```python
from build123d import *

# Parameters (mm, degrees)
F3_DEPTH = 35.967948
F5_COUNT = 3
F5_ANGLE = 240
F9_COUNT = 3
F9_ANGLE = 240


with BuildPart() as f1:
    # F0 (on Front) → F1 (revolve)
    with BuildSketch(Plane.XZ):
        with BuildLine():
            Line((-35.966948, -26.884749), (-31.12, -26.884749))
            Line((-31.12, -26.884749), (-31.12, -6.884749))
            Line((-31.12, -6.884749), (-25, 13.115251))
            Line((-25, 13.115251), (-6.375, 13.115251))
            Line((-6.375, 13.115251), (-6.375, 33.962199))
            Line((-6.375, 33.962199), (-11.221948, 33.962199))
            ThreePointArc((-11.221948, 33.962199), (-15.908239, 22.64849), (-27.221948, 17.962199))
            Line((-27.221948, 17.962199), (-28.585629, 17.962199))
            Line((-28.585629, 17.962199), (-35.966948, -6.159757))
            Line((-35.966948, -6.159757), (-35.966948, -26.884749))
        make_face()
    revolve(axis=Axis((0, 0, 3.115251), (0, 0, -1)))

    # F2 (on Front) → F3 (cut, through all)
    with BuildSketch(Plane.XZ):
        with BuildLine():
            ThreePointArc((5.600963, 5.956731), (0.100963, 11.456731), (-5.399037, 5.956731))
            Line((-5.399037, 5.956731), (5.600963, 5.956731))
        make_face()
        with BuildLine():
            Line((5.600963, 5.956731), (-5.399037, 5.956731))
            ThreePointArc((-5.399037, 5.956731), (0.100963, 0.456731), (5.600963, 5.956731))
        make_face()
    extrude(amount=-F3_DEPTH, mode=Mode.SUBTRACT)


with BuildPart() as f5_1:
    # F5: instance of F1
    add(f1.part.rotate(Axis((0, 0, 22.867789), (0, 0, 1)), 1 * F5_ANGLE / (F5_COUNT - 1)))


with BuildPart() as f5_2:
    # F5: instance of F1
    add(f1.part.rotate(Axis((0, 0, 22.867789), (0, 0, 1)), 2 * F5_ANGLE / (F5_COUNT - 1)))


with BuildPart() as f9_1:
    # F9: instance of F1
    add(f1.part.rotate(Axis((0, 0, 23.663558), (0, 0, 1)), 1 * F9_ANGLE / (F9_COUNT - 1)))


with BuildPart() as f9_2:
    # F9: instance of F1
    add(f1.part.rotate(Axis((0, 0, 23.663558), (0, 0, 1)), 2 * F9_ANGLE / (F9_COUNT - 1)))


solid = f1.part
```
Input: part model. Units: mm. Frame: model coordinates. A direction names the side the tool comes from. Coordinates: 2 decimals unless noted, no trailing zeros. Loops run counter-clockwise (first coordinate to the right, second up) from the corner with the lowest first, then second, coordinate; pieces in that order, holes last. Notation, with made-up numbers: M 42,37 L 53,37 A18 ccw 53,64 Z; hole C 2,33.25 d6. An arc over 180 degrees is marked long. One line per item, written item: value.
(1) Section C-C (z = -19). Output: boundary loops of the cut face in (x, y), and give its area (3 significant figures).
Filled in:
outline: C 0,0 d71.93; hole C 0,0 d62.24
area: 1,020 mm^2
(2) Section D-D (z = 30.5). Output: boundary loops of the cut face in (x, y) (3 decimals).
Filled in:
outline: C 0,0 d23.202; hole C 0,0 d12.75
(3) Line query: line 1 along Y through (x, z) = (0, -14); line 2 along X through (y, z) = (-1.5, -9.5); line 3 along Y through (x, z) = (-2, -11). Output: solid intervals per line, ascending. Write a range as from..to.
Filled in:
line 1: -35.97..-31.12, 31.12..35.97
line 2: -35.94..-31.08, 31.08..35.94
line 3: -35.91..-31.06, 31.06..35.91
(4) Pull-direction query (Y, two-part tool) for faces 1 (the flat face through (-5, -5, 13.115)), 2 (the conical face through (6.47, -29.16, 13.77)), 3 (the flat face through (5, -5, 33.962)); classes: +Y half, -Y half, draft (parallel to the pull), parting line (faces both ways), or undercut.
Filled in:
face 1: undercut
face 2: parting line
face 3: draft
(5) Reachability of faces 4 (the flat face through (25.3, -10.5, 17.962)), 5 (the cylindrical face through (4.47, 29.67, 9.3)), 6 (the cylindrical face through (6.75, -30.38, -16.74)) from +Z, -Z, +X, -X, +Y, -Y: full face, straight path, thin tool, end or side. Return the list, or none.
Filled in:
face 4: +Z
face 5: +Y
face 6: -Z
(6) Section B-B (y = 0). Output: boundary loops of the cut face in (x, z) (3 decimals).
Filled in:
outline: M -35.967,-26.885 L -31.12,-26.885 L -31.12,-6.885 L -25,13.115 L -6.375,13.115 L -6.375,33.962 L -11.222,33.962 A16 cw -27.222,17.962 L -28.586,17.962 L -35.967,-6.16 Z; M 6.375,13.115 L 25,13.115 L 31.12,-6.885 L 31.12,-26.885 L 35.967,-26.885 L 35.967,-6.16 L 28.586,17.962 L 27.222,17.962 A16 cw 11.222,33.962 L 6.375,33.962 Z
(7) Pin query (flat end, axial travel): pin 1 (1.5 mm diameter, centred on x = 20.5, z = -6.5, fed in from +Y); pin 2 (1.5 mm diameter, centred on x = -19.5, z = 9, fed in from -Y); pin 3 (8 mm diameter, centred on x = -22, z = -16.5, fed in from -Y). Return the tip coordinate at first contact, or that it passes through.
Filled in:
pin 1: y = 30.06
pin 2: y = -25.17
pin 3: y = -31.14
(8) Section A-A (x = 0). Output: boundary loops of the cut face in (y, z) (3 decimals), and give its area (3 significant figures).
Filled in:
outline: M -35.967,-26.885 L -31.12,-26.885 L -31.12,-6.885 L -25,13.115 L -6.375,13.115 L -6.375,33.962 L -11.222,33.962 A16 cw -27.222,17.962 L -28.586,17.962 L -35.967,-6.16 Z; M 6.375,13.115 L 25,13.115 L 25.508,11.456 L 30.577,11.456 L 28.586,17.962 L 27.222,17.962 A16 cw 11.222,33.962 L 6.375,33.962 Z; M 28.873,0.458 L 31.12,-6.885 L 31.12,-26.885 L 35.967,-26.885 L 35.967,-6.16 L 33.942,0.458 Z
area: 828 mm^2
